```python
from build123d import *

# Parameters (mm, degrees)
F0_R     = 5
F1_DEPTH = 25
F2_R     = 7.5
F2_R_2   = 5
F3_DEPTH = 25


with BuildPart() as f1:
    # F0 (on Top) → F1 (new body)
    with BuildSketch(Plane.XY):
        with BuildLine():
            Line((4.2, -30), (12.5, -30))
            Line((12.5, -30), (12.5, 30))
            Line((12.5, 30), (4.2, 30))
            Line((4.2, 30), (4.2, 15))
            ThreePointArc((4.2, 15), (0, 10.8), (-4.2, 15))
            Line((-4.2, 15), (-4.2, 30))
            Line((-4.2, 30), (-12.5, 30))
            Line((-12.5, 30), (-12.5, -30))
            Line((-12.5, -30), (-4.2, -30))
            Line((-4.2, -30), (-4.2, -15))
            ThreePointArc((-4.2, -15), (0, -10.8), (4.2, -15))
            Line((4.2, -15), (4.2, -30))
        make_face()
        Circle(F0_R, mode=Mode.SUBTRACT)
    extrude(amount=F1_DEPTH)

    # F2 (on face) → F3 (join)
    with BuildSketch(Plane.XY.offset(25)):
        Circle(F2_R)
        Circle(F2_R_2, mode=Mode.SUBTRACT)
    extrude(amount=F3_DEPTH)


solid = f1.part
```
Geometry: final body of the model. Coordinates: model frame, mm. A direction names the side the tool comes from. Coordinates: 2 decimals unless noted, no trailing zeros. Write each loop counter-clockwise with the first axis right and the second up, starting at its lowest first coordinate (ties: lowest second). Pieces come first, ordered by that corner, then holes. Notation, with made-up numbers: M 85.25,57.5 L 122.25,57.5 A37 ccw 122.25,95.5 Z; hole C 2.25,74.25 d10. An arc over 180 degrees is marked long. Answer as CSV lines item,"result". Start each with the question number.
Q1. Pin query (flat end, axial travel): P1, Ø4, axis at x = 4, y = 7.5, coming from the +Z side; P2, Ø3, axis at x = -8, z = 33.5, coming from the +Y side; P3, Ø12, axis at y = -6.5, z = 44.5, coming from the +X side; P4, Ø2, axis at x = -4, y = -13.5, coming from the +Z side. Return the tip coordinate at first contact, or that it passes through.
Q2. Cut plane C-C on x = 0. Return the cut outline in (y, z).
Q3. Cut plane D-D on y = -16.5. Return the cut outline in (x, z).
Q4. Cut plane B-B on z = 18. Return the cut outline in (x, y).
Q5. Cut plane A-A on y = 0. Return the cut outline in (x, z).
Q6. Mould query, pull axis X, two halves, no side actions, for faces 4 (the flat face through (4.2, 23, 12)), 5 (the flat face through (-12.5, 0, 12)), 6 (the flat face through (8, 30, 12)). Classes: released by +X, released by -X, zero draft, split by the parting line, or undercut.
Q7. Reachability of faces 1 (the cylindrical face through (-7.493, 0.33, 37.325)), 2 (the flat face through (-4.2, -23, 12)), 3 (the flat face through (-4.2, 22, 12)) from +Z, -Z, +X, -X, +Y, -Y: full face, straight path, thin tool, end or side. Return the list, or none.
Q8. Line query: line 1 (Y direction, x = -0.25, z = 38); line 2 (X direction, y = 16, z = 8); line 3 (Y direction, x = 0, z = 21.5). Output: solid intervals per line, ascending. Write a range as from..to.
Findings below:
1,P1,"stops at z = 50"
1,P2,"stops at y = 3.74"
1,P3,"stops at x = 7.48"
1,P4,"stops at z = 25"
2,outline,"M -10.8,0 L -5,0 L -5,50 L -7.5,50 L -7.5,25 L -10.8,25 Z; M 5,0 L 10.8,0 L 10.8,25 L 7.5,25 L 7.5,50 L 5,50 Z"
3,outline,"M -12.5,0 L -4.2,0 L -4.2,25 L -12.5,25 Z; M 4.2,0 L 12.5,0 L 12.5,25 L 4.2,25 Z"
4,outline,"M -12.5,-30 L -4.2,-30 L -4.2,-15 A4.2 cw 4.2,-15 L 4.2,-30 L 12.5,-30 L 12.5,30 L 4.2,30 L 4.2,15 A4.2 cw -4.2,15 L -4.2,30 L -12.5,30 Z; hole C 0,0 d10"
5,outline,"M -12.5,0 L -5,0 L -5,50 L -7.5,50 L -7.5,25 L -12.5,25 Z; M 5,0 L 12.5,0 L 12.5,25 L 7.5,25 L 7.5,50 L 5,50 Z"
6,face 4,"undercut"
6,face 5,"released by -X"
6,face 6,"zero draft"
7,face 1,"+Z"
7,face 2,"+Z, -Z, -Y"
7,face 3,"+Z, -Z, +Y"
8,line 1,"y = -7.5..-4.99, 4.99..7.5"
8,line 2,"x = -12.5..-4.2, 4.2..12.5"
8,line 3,"y = -10.8..-5, 5..10.8"
